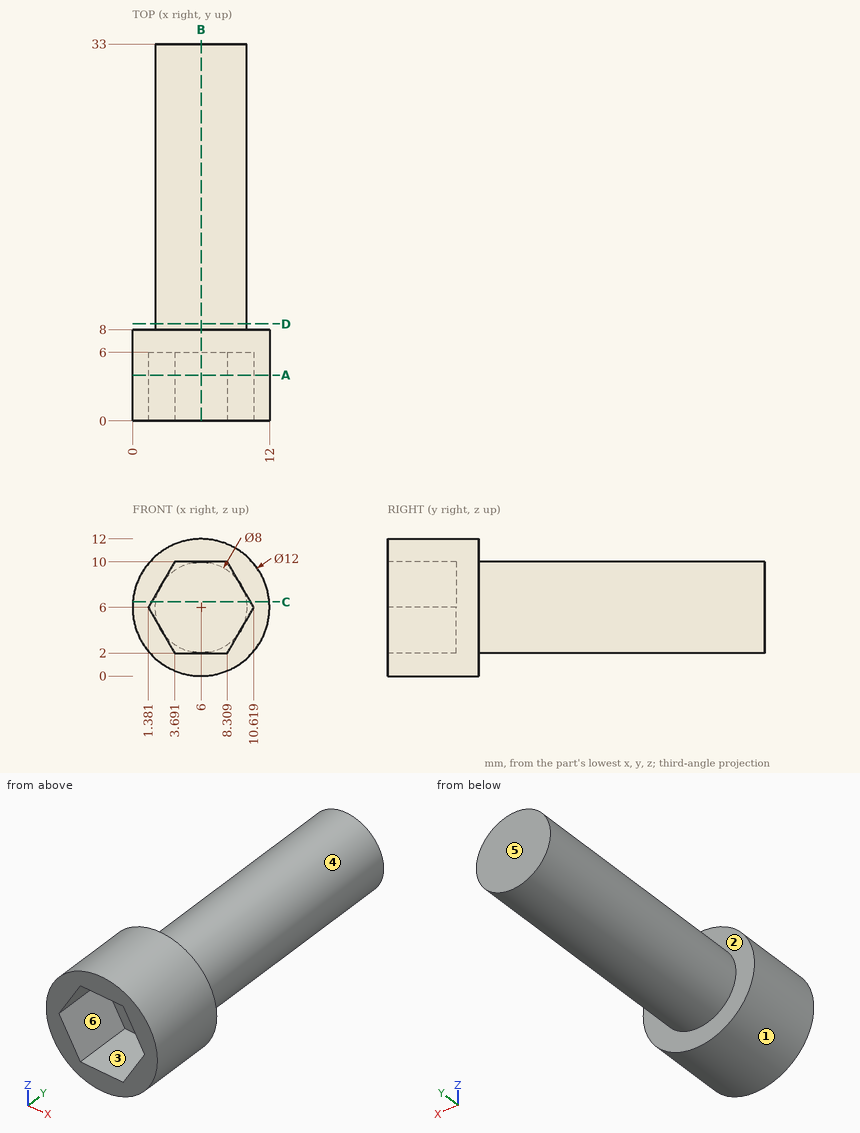
Drawing for the job (mm, zero at the part's lowest x, y, z). A direction names the side the tool comes from. Give positions to 0.01 mm unless a question says otherwise; leave off trailing zeros. Order: outer loops, then holes, each group sorted by start corner. A loop starts at its lowest first (then second) coordinate and runs counter-clockwise, first axis right, second up. Notation, with made-up numbers: M -40,41.25 L -36,41.25 A26 cw -36,64.25 Z; hole C 27,46 d9. An arc over 180 degrees is marked long. Put each result on its own line as item: value.
Item 1: Slice it at C-C, the plane z = 6.5. Write the cut outline in (x, y), plus the area to 3 significant figures.
From the geometry:
outline: M 0.02,0 L 1.67,0 L 1.67,6 L 10.33,6 L 10.33,0 L 11.98,0 L 11.98,8 L 9.97,8 L 9.97,33 L 2.03,33 L 2.03,8 L 0.02,8 Z
area: 242 mm2
Item 2: Slice it at D-D, the plane y = 8.5. Write the cut outline in (x, z).
From the geometry:
outline: C 6,6 d8
Item 3: Two-plate mould, pull along Z, no slides. Class the marked faces 4, 5 and 6: +Z half, -Z half, draft (parallel to the pull), parting line (faces both ways), or undercut.
From the geometry:
face 4: parting line
face 5: draft
face 6: undercut
Item 4: Slice it at A-A, the plane y = 4. Write the cut outline in (x, z).
From the geometry:
outline: C 6,6 d12; hole M 1.38,6 L 3.69,2 L 8.31,2 L 10.62,6 L 8.31,10 L 3.69,10 Z
Item 5: Flat gauge pins, fed straight in: pin 1 Ø4 at (y, z) = (19, 8) entering from +X; pin 2 Ø4 at (x, z) = (4.5, 7) entering from -Y. Where does each tip first touch, or does it go through?
From the geometry:
pin 1: stops at x = 10
pin 2: stops at y = 6
Item 6: Slice it at B-B, the plane x = 6. Write the cut outline in (y, z), plus the area to 3 significant figures.
From the geometry:
outline: M 0,0 L 8,0 L 8,2 L 33,2 L 33,10 L 8,10 L 8,12 L 0,12 L 0,10 L 6,10 L 6,2 L 0,2 Z
area: 248 mm2
Item 7: 3-axis set-ups, long thin cutter, end or side, ignore diameter. For the marked faces 1, 2 and 3: which of +Z, -Z, +X, -X, +Y, -Y reach the whole face in a straight line?
From the geometry:
face 1: +Y, -Y
face 2: +Y
face 3: -Y
Item 8: Probe line 1 (Y direction, x = 6.5, z = 6.25); line 2 (X direction, y = 28, z = 5.75); line 3 (Y direction, x = 10.5, z = 5). List the from-to ranges inside material, lowest first. Write a range as [from, to].
From the geometry:
line 1: y = [6, 33]
line 2: x = [2.01, 9.99]
line 3: y = [0, 8]
